Check sheet for the drawn part. Datum: minimum x, y, z corner. Units: mm. A direction names the side the tool comes from. Round coordinates to 2 decimals unless told otherwise and drop trailing zeros. Write each loop counter-clockwise with the first axis right and the second up, starting at its lowest first coordinate (ties: lowest second). Pieces come first, ordered by that corner, then holes. Notation, with made-up numbers: (7, -17) - (50, -17) arc R15 cw to (50, 3) - close; hole circle Ø10 at (56, -32.75). An arc over 180 degrees is marked (long way). Answer as a JSON object with one key per item and string values.
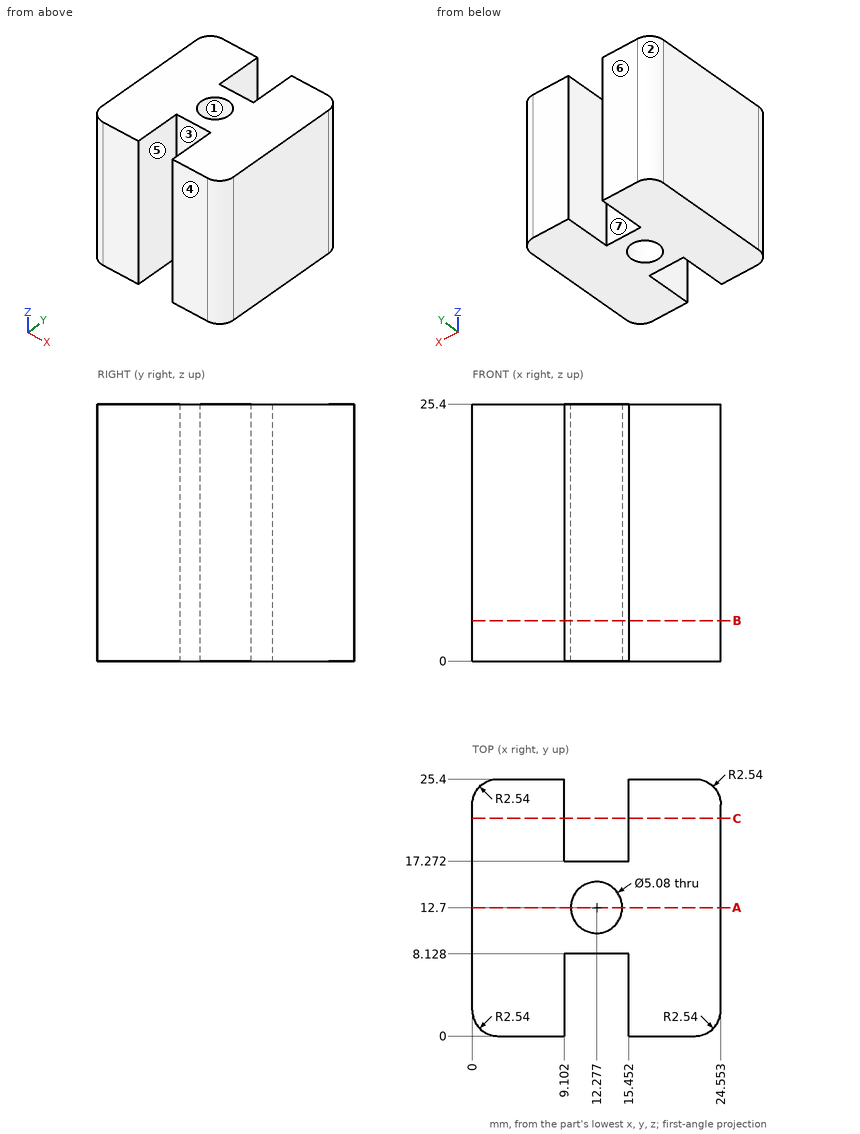
1. Cross-section at A-A (y = 12.7). Record the boundary of the cut face in (x, z).
Completed:
{"outline": "(0, 0) - (9.74, 0) - (9.74, 25.4) - (0, 25.4) - close; (14.82, 0) - (24.55, 0) - (24.55, 25.4) - (14.82, 25.4) - close"}
2. Cross-section at B-B (z = 4). Record the boundary of the cut face in (x, y), plus the area to 3 significant figures.
Completed:
{"outline": "(0, 2.54) arc R2.54 ccw to (2.54, 0) - (9.1, 0) - (9.1, 8.13) - (15.45, 8.13) - (15.45, 0) - (22.01, 0) arc R2.54 ccw to (24.55, 2.54) - (24.55, 22.86) arc R2.54 ccw to (22.01, 25.4) - (15.45, 25.4) - (15.45, 17.27) - (9.1, 17.27) - (9.1, 25.4) - (2.54, 25.4) arc R2.54 ccw to (0, 22.86) - close; hole circle Ø5.08 at (12.28, 12.7)", "area": "495 mm^2"}
3. Access from +Z, -Z, +X, -X, +Y, -Y to the whole of each face (thin tool, end or side, straight path). Record for the marked faces 5, 6 and 7.
Completed:
{"face 5": "+Z, -Z, -Y", "face 6": "+Z, -Z, +X, -X, +Y", "face 7": "+Z, -Z, +Y"}
4. Cross-section at C-C (y = 21.5). Record the boundary of the cut face in (x, z).
Completed:
{"outline": "(0, 0) - (9.1, 0) - (9.1, 25.4) - (0, 25.4) - close; (15.45, 0) - (24.55, 0) - (24.55, 25.4) - (15.45, 25.4) - close"}
5. Go/stop test with flat-tipped pins: pin 1 (1.5 mm diameter, centred on x = 13.5, y = 14.5, fed in from -Z); pin 2 (1.9 mm diameter, centred on x = 11, z = 10.5, fed in from -Y). Record where each tip stops, or that it passes through.
Completed:
{"pin 1": "stops at z = 0", "pin 2": "stops at y = 8.13"}
6. Mould release check, pull along X, two halves, no side actions. Record for the marked faces 1, 2, 3 and 4: released by +X, released by -X, zero draft, split by the parting line, or undercut.
Completed:
{"face 1": "undercut", "face 2": "released by -X", "face 3": "undercut", "face 4": "zero draft"}
7. Material ranges on probe 1 along X at (y, z) = (5, 16.5); probe 2 along Y at (x, z) = (11.25, 1); probe 3 along Y at (x, z) = (15, 14.5), recorded low to high. Write a range as from..to.
Completed:
{"probe 1": "x = 0..9.1, 15.45..24.55", "probe 2": "y = 8.13..10.38, 15.02..17.27", "probe 3": "y = 8.13..17.27"}
